Work out the finished part from the listing and answer in its coordinate system (mm). A direction names the side the tool comes from. Round coordinates to 2 decimals unless told otherwise and drop trailing zeros. Write each loop counter-clockwise with the first axis right and the second up, starting at its lowest first coordinate (ties: lowest second). Pieces come first, ordered by that corner, then holes. Notation, with made-up numbers: (16.5, 22) -> (68.5, 22) arc R7 ccw to (68.5, 35) -> close; hole circle Ø5 at (-19, -3). An arc over 180 degrees is marked (long way). One line per item, written item: value.
```python
from build123d import *

# Parameters (mm, degrees)
F1_DEPTH      = 5
F2_R          = 1.5
F3_DEPTH      = 2.501
F3_DEPTH_BACK = 7.501


with BuildPart() as f1:
    # F0 (on Front) → F1 (new body, symmetric)
    with BuildSketch(Plane.XZ):
        Polygon((-5, 0), (0, 0), (0, 5), (-2.5, 5), (-2.5, 10), (-5, 10), align=None)
        Polygon((0, 5), (0, 0), (5, 0), (5, 10), (2.5, 10), (2.5, 5), align=None)
    extrude(amount=F1_DEPTH, both=True)

    # F2 (on face) → F3 (cut, two sides)
    with BuildSketch(Plane.YZ.offset(-2.5)) as f3_sk:
        with Locations((0, 7.5)):
            Circle(F2_R)
    extrude(amount=-F3_DEPTH, mode=Mode.SUBTRACT)
    extrude(f3_sk.sketch, amount=F3_DEPTH_BACK, mode=Mode.SUBTRACT)


solid = f1.part
```
(1) Find section C-C on z = 7.5. Give the vertices of the cut face in (x, y), plus the area to 3 significant figures.
Reported:
outline: (-5, -5) -> (-2.5, -5) -> (-2.5, -1.5) -> (-5, -1.5) -> close; (-5, 1.5) -> (-2.5, 1.5) -> (-2.5, 5) -> (-5, 5) -> close; (2.5, -5) -> (5, -5) -> (5, -1.5) -> (2.5, -1.5) -> close; (2.5, 1.5) -> (5, 1.5) -> (5, 5) -> (2.5, 5) -> close
area: 35.0 mm2
(2) For a pull along Y with two mould halves and no side action, classify faces 3 (the face through (-4, 0, 6)), 4 (the face through (0, -5, 4)), 5 (the face through (-5, 0, 5)) as pulls with the +Y half, pulls with the -Y half, needs draft (parallel to the pull), parting line crosses it, or undercut.
Reported:
face 3: undercut
face 4: pulls with the -Y half
face 5: needs draft
(3) A tool of negligible diameter and unlimited length cuts with its end or side. For faces 1 (the face through (0, 5, 4)), 2 (the face through (-2.5, -1, 6)), from which of +Z, -Z, +X, -X, +Y, -Y can it reach the whole face along a straight path? Write none if from no direction.
Reported:
face 1: +Z, -Z, +X, -X, +Y
face 2: +Z, +Y, -Y
(4) Find section B-B on y = 0. Give the vertices of the cut face in (x, z).
Reported:
outline: (-5, 0) -> (5, 0) -> (5, 6) -> (2.5, 6) -> (2.5, 5) -> (-2.5, 5) -> (-2.5, 6) -> (-5, 6) -> close; (-5, 9) -> (-2.5, 9) -> (-2.5, 10) -> (-5, 10) -> close; (2.5, 9) -> (5, 9) -> (5, 10) -> (2.5, 10) -> close
(5) Find section D-D on x = 2.75. Give the vertices of the cut face in (y, z), plus the area to 3 significant figures.
Reported:
outline: (-5, 0) -> (5, 0) -> (5, 10) -> (-5, 10) -> close; hole circle Ø3 at (0, 7.5)
area: 92.9 mm2
(6) Flat-ended cylindrical pins translate along their axes: pin 1 Ø2.5 at (y, z) = (0, 7.5) entering from +X; pin 2 Ø2.5 at (x, y) = (0.5, 0.5) entering from +Z. Find the tip coordinate at first contact, or state that the pin passes through.
Reported:
pin 1: passes through
pin 2: stops at z = 5
(7) Consider probe 1 along X at (y, z) = (4, 6.5); probe 2 along Y at (x, z) = (4.4, 7.5); probe 3 along Z at (x, y) = (-3.4, 0). Determine where each line is inside the solid, lowest interval first.
Reported:
probe 1: x = -5 to -2.5, 2.5 to 5
probe 2: y = -5 to -1.5, 1.5 to 5
probe 3: z = 0 to 6, 9 to 10
(8) Find section A-A on z = 5.75. Give the vertices of the cut face in (x, y).
Reported:
outline: (-5, -5) -> (-2.5, -5) -> (-2.5, 5) -> (-5, 5) -> close; (2.5, -5) -> (5, -5) -> (5, 5) -> (2.5, 5) -> close
